Source: CAD feature listing. Evaluate the final solid. Frame: model axes, mm. Face numbers are marked on the shaded views. A direction names the side the tool comes from. Round coordinates to 2 decimals unless told otherwise and drop trailing zeros. Answer in a Markdown table with one row per item.
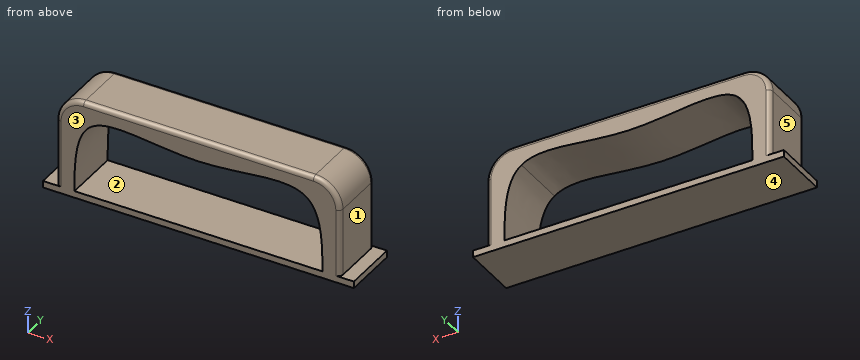
from build123d import *

# Parameters (mm, degrees)
F0_W     = 6
F0_H     = 3
F1_DEPTH = 25
F2_R     = 12
F3_R     = 2


with BuildPart() as f1:
    # F0 (on Front) → F1 (new body)
    with BuildSketch(Plane.XZ):
        with BuildLine():
            add(Edge.make_bspline(
                [(-55, 0), (-55.0076209993, 1.0009689247), (-55.0152419987, 2.0019378493), (-55.0204363014, 3)],
                knots=[0, 0, 0, 0, 0.0157183213, 0.0157183213, 0.0157183213, 0.0157183213], degree=3))
            Line((-55, 0), (55, 0))
            add(Edge.make_bspline(
                [(55.0204363014, 3), (55.0152419987, 2.0019378493), (55.0076209993, 1.0009689247), (55, 0)],
                knots=[0.9842816787, 0.9842816787, 0.9842816787, 0.9842816787, 1, 1, 1, 1], degree=3))
            Line((55.0204363014, 3), (-55.0204363014, 3))
        make_face()
        with BuildLine():
            Line((-63, 0), (-55, 0))
            add(Edge.make_bspline(
                [(-55, 0), (-55.0076209993, 1.0009689247), (-55.0152419987, 2.0019378493), (-55.0204363014, 3)],
                knots=[0, 0, 0, 0, 0.0157183213, 0.0157183213, 0.0157183213, 0.0157183213], degree=3))
            Line((-55.0204363014, 3), (-63, 3))
            Line((-63, 3), (-63, 0))
        make_face()
        with BuildLine():
            add(Edge.make_bspline(
                [(55.0204363014, 3), (55.0152419987, 2.0019378493), (55.0076209993, 1.0009689247), (55, 0)],
                knots=[0.9842816787, 0.9842816787, 0.9842816787, 0.9842816787, 1, 1, 1, 1], degree=3))
            Line((55, 0), (63, 0))
            Line((63, 0), (63, 3))
            Line((63, 3), (55.0204363014, 3))
        make_face()
        with BuildLine():
            Line((-63, 3), (-55.0204363014, 3))
            add(Edge.make_bspline(
                [(-55.0204363014, 3), (-55.0920234657, 16.7551548981), (-54.7026845561, 29.9581979592), (-47.5, 35)],
                knots=[0.0157183213, 0.0157183213, 0.0157183213, 0.0157183213, 0.2323460581, 0.2323460581, 0.2323460581, 0.2323460581], degree=3))
            add(Edge.make_bspline(
                [(-47.5, 35), (-38.6007383304, 41.229387848), (-19.3003691017, 34.9999999795), (1.271e-07, 35)],
                knots=[0.2323460581, 0.2323460581, 0.2323460581, 0.2323460581, 0.5, 0.5, 0.5, 0.5], degree=3))
            add(Edge.make_bspline(
                [(1.271e-07, 35), (19.3003692287, 35.0000000205), (38.60073836, 41.2293878575), (47.5000000137, 35.0000000044)],
                knots=[0.5, 0.5, 0.5, 0.5, 0.7676539419, 0.7676539419, 0.7676539419, 0.7676539419], degree=3))
            add(Edge.make_bspline(
                [(47.5, 35), (54.7026845561, 29.9581979592), (55.0920234657, 16.7551548981), (55.0204363014, 3)],
                knots=[0.7676539419, 0.7676539419, 0.7676539419, 0.7676539419, 0.9842816787, 0.9842816787, 0.9842816787, 0.9842816787], degree=3))
            Line((55.0204363014, 3), (63, 3))
            Line((63, 3), (63, 45))
            Line((63, 45), (-63, 45))
            Line((-63, 45), (-63, 3))
        make_face()
        with Locations((-66, 1.5)):
            Rectangle(F0_W, F0_H)
        with Locations((66, 1.5)):
            Rectangle(F0_W, F0_H)
    extrude(amount=F1_DEPTH)

    # F2
    f2_edges = [f1.edges().sort_by_distance(p)[0] for p in [
        (-63, -12.5, 45),
        (63, -12.5, 45),
    ]]
    fillet(f2_edges, radius=F2_R)

    # F3
    f3_edges = [f1.edges().sort_by_distance(p)[0] for p in [
        (0, 0, 45),
        (-59.485281, 0, 41.485281),
        (-63, 0, 18),
        (59.485281, 0, 41.485281),
        (63, 0, 18),
        (-63, -25, 18),
        (-59.485281, -25, 41.485281),
        (0, -25, 45),
        (59.485281, -25, 41.485281),
        (63, -25, 18),
    ]]
    fillet(f3_edges, radius=F3_R)


solid = f1.part
Q1. Material intervals for probe 1 along X at (y, z) = (-5.25, 8.5); probe 2 along Z at (x, y) = (-7, -17.5); probe 3 along Z at (x, y) = (18.5, -14.25), sorted ascending.
Solutions:
| item | result |
|---|---|
| probe 1 | x = -63 to -55.01, 55.01 to 63 |
| probe 2 | z = 0 to 3, 35.24 to 45 |
| probe 3 | z = 0 to 3, 36.34 to 45 |
Q2. Pull-direction query (X, two-part tool) for the marked faces 1, 2 and 3; classes: pulls with the +X half, pulls with the -X half, needs draft (parallel to the pull), parting line crosses it, or undercut.
Solutions:
| item | result |
|---|---|
| face 1 | pulls with the +X half |
| face 2 | undercut |
| face 3 | needs draft |
Q3. Access query for the marked faces 4 and 5. Directions: +Z, -Z, +X, -X, +Y, -Y. A direction counts if a zero-diameter tool reaches every point of the face in a straight line with its end or side. Return the directions, or none.
Solutions:
| item | result |
|---|---|
| face 4 | -Z, +X, -X, +Y, -Y |
| face 5 | +Z, -X, +Y, -Y |
Q4. Contact query for flat-ended pins moving along their axis: pin 1 Ø10 at (y, z) = (-21, 17.5) entering from +X; pin 2 Ø9 at (x, y) = (-66.5, -15) entering from +Z; pin 3 Ø6.5 at (x, y) = (65, -9) entering from +Z. Output: stop coordinate, or through.
Solutions:
| item | result |
|---|---|
| pin 1 | stops at x = 63 |
| pin 2 | stops at z = 37.8 |
| pin 3 | stops at z = 38.33 |
